Build history of the part. All positions in model axes, mm. A direction names the side the tool comes from. Give positions to 0.01 mm unless a question says otherwise; leave off trailing zeros. Write each loop counter-clockwise with the first axis right and the second up, starting at its lowest first coordinate (ties: lowest second). Pieces come first, ordered by that corner, then holes. Notation, with made-up numbers: (59, -10.75) -> (98, -10.75) arc R31 cw to (98, 20.25) -> close; hole circle Ø10 at (-30.5, 19). An arc over 180 degrees is marked (long way). Put each result on its own line as item: value. Start each with the question number.
Item 1: Flat gauge pins, fed straight in: pin 1 Ø5 at (x, y) = (-2, 12) entering from -Z; pin 2 Ø3 at (y, z) = (7.5, -3.5) entering from -X. Where does each tip first touch, or does it go through?
Item 2: Slice it at B-B, the plane x = 0. List the corners of the cut face in (y, z), plus the area to 3 significant figures.
Item 3: Slice it at C-C, the plane y = 15.5. List the corners of the cut face in (x, z).
Item 4: Slice it at D-D, the plane z = -5.5. List the corners of the cut face in (x, y), plus the area to 3 significant figures.
Item 5: Drill centre lines: line 1 along Y through (x, z) = (-4.5, 4); line 2 along X through (y, z) = (16, 0.25); line 3 along Z through (x, y) = (-3, 5). Where is each one in solid material? Low to high.
Item 6: Slice it at A-A, the plane z = 0. List the corners of the cut face in (x, y).
Item 7: Tool access for faces 1 (the flat face through (-5, 21.65, 0)), 2 (the cylindrical face through (-3.905, 5.916, -0.867)), 3 (the flat face through (0, 0, 0)): list every direction of +Z, -Z, +X, -X, +Y, -Y with a clear straight run to the whole face (end or side of a thin tool).
```python
from build123d import *

# Parameters (mm, degrees)
SKETCH_1_R      = 4
EXTRUDE_1_DEPTH = 12
SKETCH_2_R      = 7
EXTRUDE_2_DEPTH = 9.65


with BuildPart() as part:
    # 草图1 → 凸台-拉伸1 (new body)
    with BuildSketch(Plane(origin=(0, 0, 0), x_dir=(1, 0, 0), z_dir=(0, 1, 0))):
        with Locations(Location((0, 0, 0), (0, 0, 270))):
            Circle(SKETCH_1_R)
    extrude(amount=EXTRUDE_1_DEPTH)

    # 草图2 → 凸台-拉伸2 (add)
    with BuildSketch(Plane(origin=(0, 12, 0), x_dir=(1, 0, 0), z_dir=(0, 1, 0))):
        with Locations(Location((0, 0, 0), (0, 0, 270))):
            Circle(SKETCH_2_R)
    extrude(amount=EXTRUDE_2_DEPTH)

    # 草图3 → 旋转1 (revolve)
    with BuildSketch(Plane(origin=(0, 21.65, 0), x_dir=(1, 0, 0), z_dir=(0, 1, 0))):
        with BuildLine():
            Line((0, 4.35), (0, -4.35))
            ThreePointArc((0, -4.35), (4.35, 0), (0, 4.35))
        make_face()
    revolve(axis=Axis((0, 21.65, -4.35), (0, 0, 1)))


solid = part.part
```
Values follow:
1. pin 1: z = -7
1. pin 2: x = -3.46
2. outline: (0, -4) -> (12, -4) -> (12, -7) -> (21.65, -7) -> (21.65, -4.35) arc R4.35 ccw to (21.65, 4.35) -> (21.65, 7) -> (12, 7) -> (12, 4) -> (0, 4) -> close
2. area: 261 mm2
3. outline: circle Ø14 at (0, 0)
4. outline: (-4.33, 12) -> (4.33, 12) -> (4.33, 21.65) -> (-4.33, 21.65) -> close
4. area: 83.6 mm2
5. line 1: 12 to 21.65
5. line 2: -7 to 7
5. line 3: -2.65 to 2.65
6. outline: (-7, 12) -> (-4, 12) -> (-4, 0) -> (4, 0) -> (4, 12) -> (7, 12) -> (7, 21.65) -> (4.35, 21.65) arc R4.35 ccw to (-4.35, 21.65) -> (-7, 21.65) -> close
7. face 1: +Y
7. face 2: -Y
7. face 3: +Z, -Z, +X, -X, -Y
